Can you work these out from the drawing? Everything is in mm from the part's minimum corner. A direction names the side the tool comes from. Coordinates: 2 decimals unless noted, no trailing zeros. Write each loop counter-clockwise with the first axis right and the second up, starting at its lowest first coordinate (ties: lowest second). Pieces come first, ordered by that corner, then holes.
(1) Imagine slicing it at B-B, the plane x = 18.7. List the corners of the cut face in (y, z) for me (3 decimals), plus the area to 3 significant figures.
(2) Thinking about a two-plate mould opening in X: for the marked faces 1, 2 and 3, which applies, released by +X, released by -X, zero draft, split by the parting line, or undercut?
(3) Imagine slicing it at A-A, the plane y = 4.5. List the corners of the cut face in (x, z) for me, plus the area to 3 significant figures.
(4) Imagine slicing it at D-D, the plane y = 26.5. List the corners of the cut face in (x, z) for me.
(5) Which directions (+Z, -Z, +X, -X, +Y, -Y) give clear straight access to the entire face, cutting with the end or side of a thin tool? Please do the marked faces 4, 5 and 6.
(6) Imagine slicing it at C-C, the plane z = 12.7. List the corners of the cut face in (x, y) for me (3 decimals), plus the area to 3 significant figures.
(7) Please list where these lines run through material, in increasing order: probe 1 along X at (y, z) = (4, 11.75); probe 2 along Y at (x, z) = (33, 7) (3 decimals); probe 3 along Y at (x, z) = (10.5, 21.75) (3 decimals).
(8) For pin 1 Ø7.5 at (x, z) = (23, 18.5) entering from -Y; pin 2 Ø2 at (y, z) = (22.5, 10.5) entering from +X; pin 3 Ø6 at (y, z) = (23.5, 21.5) entering from +X, each with a flat end and sliding along its axis, tell me the tip position at first contact or that it passes through.
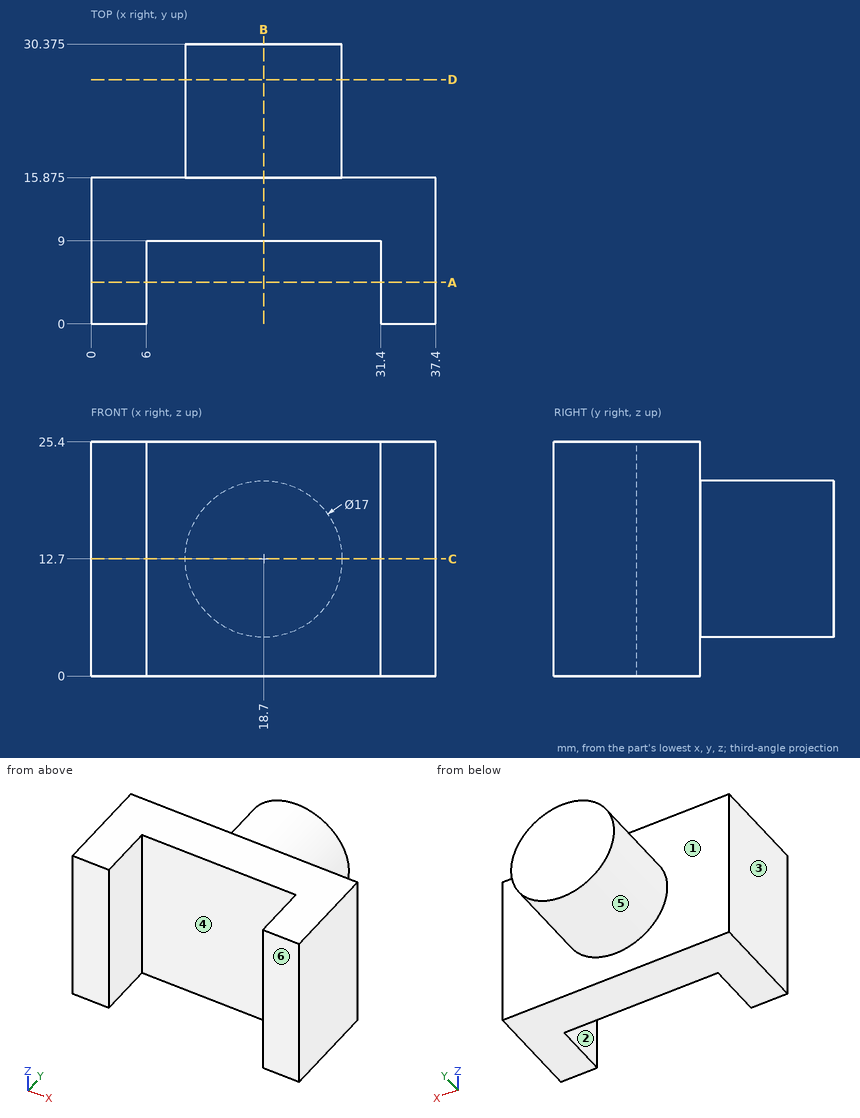
Recorded:
1. outline: (9, 0) - (15.875, 0) - (15.875, 4.2) - (30.375, 4.2) - (30.375, 21.2) - (15.875, 21.2) - (15.875, 25.4) - (9, 25.4) - close
1. area: 421 mm2
2. face 1: zero draft
2. face 2: undercut
2. face 3: released by -X
3. outline: (0, 0) - (6, 0) - (6, 25.4) - (0, 25.4) - close; (31.4, 0) - (37.4, 0) - (37.4, 25.4) - (31.4, 25.4) - close
3. area: 305 mm2
4. outline: circle Ø17 at (18.7, 12.7)
5. face 4: +Z, -Z, -Y
5. face 5: +Y
5. face 6: +Z, -Z, +X, -X, -Y
6. outline: (0, 0) - (6, 0) - (6, 9) - (31.4, 9) - (31.4, 0) - (37.4, 0) - (37.4, 15.875) - (27.2, 15.875) - (27.2, 30.375) - (10.2, 30.375) - (10.2, 15.875) - (0, 15.875) - close
6. area: 612 mm2
7. probe 1: x = 0 to 6, 31.4 to 37.4
7. probe 2: y = 0 to 15.875
7. probe 3: y = 9 to 15.875
8. pin 1: stops at y = 9
8. pin 2: stops at x = 27.11
8. pin 3: stops at x = 24.91
